from build123d import *

# Parameters (mm, degrees)
BOSS_EXTRUDE1_DEPTH            = 1.6
BOSS_EXTRUDE2_DEPTH            = 0.1
M2_HOLE1_FIXINGSTRUCTURE_D     = 2.4
M2_HOLE1_FIXINGSTRUCTURE_DEPTH = 200
M2_HOLE1_FIXINGSTRUCTURE_TIP   = 0.721032743
SKETCH4_W                      = 30
SKETCH4_H                      = 15
CUT_EXTRUDE1_DEPTH             = 1.7


with BuildPart() as part:
    # Sketch1 → Boss-Extrude1 (new body)
    with BuildSketch(Plane.XY):
        with BuildLine():
            Line((-34, 44), (-34, 38))
            ThreePointArc((-34, 38), (-34.146446609, 37.646446609), (-34.5, 37.5))
            Line((-34.5, 37.5), (-40.5, 37.5))
            ThreePointArc((-40.5, 37.5), (-40.853553391, 37.353553391), (-41, 37))
            Line((-41, 37), (-41, -37))
            ThreePointArc((-41, -37), (-40.853553391, -37.353553391), (-40.5, -37.5))
            Line((-40.5, -37.5), (-34.5, -37.5))
            ThreePointArc((-34.5, -37.5), (-34.146446609, -37.646446609), (-34, -38))
            Line((-34, -38), (-34, -44))
            ThreePointArc((-34, -44), (-33.853553391, -44.353553391), (-33.5, -44.5))
            Line((-33.5, -44.5), (33.5, -44.5))
            ThreePointArc((33.5, -44.5), (33.853553391, -44.353553391), (34, -44))
            Line((34, -44), (34, -38))
            ThreePointArc((34, -38), (34.146446609, -37.646446609), (34.5, -37.5))
            Line((34.5, -37.5), (40.5, -37.5))
            ThreePointArc((40.5, -37.5), (40.853553391, -37.353553391), (41, -37))
            Line((41, -37), (41, 37))
            ThreePointArc((41, 37), (40.853553391, 37.353553391), (40.5, 37.5))
            Line((40.5, 37.5), (34.5, 37.5))
            ThreePointArc((34.5, 37.5), (34.146446609, 37.646446609), (34, 38))
            Line((34, 38), (34, 44))
            ThreePointArc((34, 44), (33.853553391, 44.353553391), (33.5, 44.5))
            Line((33.5, 44.5), (-33.5, 44.5))
            ThreePointArc((-33.5, 44.5), (-33.853553391, 44.353553391), (-34, 44))
        make_face()
    extrude(amount=BOSS_EXTRUDE1_DEPTH)

    # Esboço1 → Boss-Extrude2 (add)
    with BuildSketch(Plane.XY.offset(1.6)):
        with BuildLine():
            Line((-29.5, -37.5), (29.5, -37.5))
            ThreePointArc((29.5, -37.5), (30.805038314, -37.308461045), (32, -36.75))
            ThreePointArc((32, -36.75), (33.194961686, -36.191538955), (34.5, -36))
            ThreePointArc((34.5, -36), (38.035533906, -34.535533906), (39.5, -31))
            Line((39.5, -31), (39.5, 31))
            ThreePointArc((39.5, 31), (38.035533906, 34.535533906), (34.5, 36))
            ThreePointArc((34.5, 36), (33.194961686, 36.191538955), (32, 36.75))
            ThreePointArc((32, 36.75), (30.805038314, 37.308461045), (29.5, 37.5))
            Line((29.5, 37.5), (-29.5, 37.5))
            ThreePointArc((-29.5, 37.5), (-30.805038314, 37.308461045), (-32, 36.75))
            ThreePointArc((-32, 36.75), (-33.194961686, 36.191538955), (-34.5, 36))
            ThreePointArc((-34.5, 36), (-38.035533906, 34.535533906), (-39.5, 31))
            Line((-39.5, 31), (-39.5, -31))
            ThreePointArc((-39.5, -31), (-38.035533906, -34.535533906), (-34.5, -36))
            ThreePointArc((-34.5, -36), (-33.194961686, -36.191538955), (-32, -36.75))
            ThreePointArc((-32, -36.75), (-30.805038314, -37.308461045), (-29.5, -37.5))
        make_face()
    extrude(amount=BOSS_EXTRUDE2_DEPTH)

    # M2 Hole1-FixingStructure
    with Locations(Plane(origin=(0, 0, 0), x_dir=(-1, 0, 0), z_dir=(0, 0, -1))):
        with Locations((-30.5, 40.5), (30.5, 40.5), (-30.5, -40.5), (30.5, -40.5)):
            Hole(M2_HOLE1_FIXINGSTRUCTURE_D / 2, depth=M2_HOLE1_FIXINGSTRUCTURE_DEPTH)
            with Locations((0, 0, -(M2_HOLE1_FIXINGSTRUCTURE_DEPTH + M2_HOLE1_FIXINGSTRUCTURE_TIP / 2))):  # 118° drill point
                Cone(0, M2_HOLE1_FIXINGSTRUCTURE_D / 2, M2_HOLE1_FIXINGSTRUCTURE_TIP, mode=Mode.SUBTRACT)

    # Sketch4 → Cut-Extrude1 (cut)
    with BuildSketch(Plane(origin=(0, 0, 0), x_dir=(-1, 0, 0), z_dir=(0, 0, -1))):
        with Locations((0, 13.4)):
            Rectangle(SKETCH4_W, SKETCH4_H)
    extrude(amount=-CUT_EXTRUDE1_DEPTH, mode=Mode.SUBTRACT)


solid = part.part
Verification items for the finished model (mm, model axes). Coordinates: 2 decimals unless noted, no trailing zeros. Order: outer loops, then holes, each group sorted by start corner. A loop starts at its lowest first (then second) coordinate and runs counter-clockwise, first axis right, second up. Notation, with made-up numbers: M 7,-17 L 16,-17 A24 cw 16,8 Z; hole C 27,33.5 d11. An arc over 180 degrees is marked long. One line per item, written item: value. Start each with the question number.
Item 1: Sectioned sample at C-C (y = -40.5). Enter the section's corners in (x, z), then the cut area to 3 significant figures.
Item 2: Scan lines: probe 1 along Y at (x, z) = (-30.5, 0.8); probe 2 along Y at (x, z) = (5.5, 0.35); probe 3 along Y at (x, z) = (-5, 1.65). Record each from-to range of solid material in increasing order.
Item 3: Sectioned sample at A-A (y = 15.5). Enter the section's corners in (x, z).
Item 4: Sectioned sample at D-D (z = 0.45). Count the separate pieces of the cut face and the enclosed holes in it, then the cut area to 3 significant figures.
Item 5: Mould release check, pull along Y, two halves, no side actions. Record for faces 1 (the flat face through (-40, 4, 1.6)), 2 (the cylindrical face through (31.15, -39.49, 0.81)): released by +Y, released by -Y, zero draft, split by the parting line, or undercut.
Item 6: Sectioned sample at B-B (x = -8). Enter the section's corners in (y, z), then the cut area to 3 significant figures.
Item 7: Gauge pin test, flat ends, axial feed: pin 1 (1.9 mm diameter, centred on x = 30.5, y = 40.5, fed in from +Z); pin 2 (0.5 mm diameter, centred on x = -36.5, z = 1, fed in from -Y); pin 3 (4 mm diameter, centred on x = 30.5, y = -40.5, fed in from +Z); pin 4 (0.5 mm diameter, centred on y = 40, z = 1, fed in from +X). Record the tip position at first contact, or that the pin passes through.
Conclusion:
1. outline: M -34,0 L -31.7,0 L -31.7,1.6 L -34,1.6 Z; M -29.3,0 L 29.3,0 L 29.3,1.6 L -29.3,1.6 Z; M 31.7,0 L 34,0 L 34,1.6 L 31.7,1.6 Z
1. area: 101 mm^2
2. probe 1: y = -44.5 to -41.7, -39.3 to 39.3, 41.7 to 44.5
2. probe 2: y = -44.5 to 5.9, 20.9 to 44.5
2. probe 3: y = -37.5 to 5.9, 20.9 to 37.5
3. outline: M -41,0 L -15,0 L -15,1.7 L -39.5,1.7 L -39.5,1.6 L -41,1.6 Z; M 15,0 L 41,0 L 41,1.6 L 39.5,1.6 L 39.5,1.7 L 15,1.7 Z
4. separate pieces: 1
4. enclosed holes: 5
4. area: 6,630 mm^2
5. face 1: zero draft
5. face 2: undercut
6. outline: M -44.5,0 L 5.9,0 L 5.9,1.7 L -37.5,1.7 L -37.5,1.6 L -44.5,1.6 Z; M 20.9,0 L 44.5,0 L 44.5,1.6 L 37.5,1.6 L 37.5,1.7 L 20.9,1.7 Z
6. area: 124 mm^2
7. pin 1: passes through
7. pin 2: stops at y = -37.5
7. pin 3: stops at z = 1.6
7. pin 4: stops at x = 34
